Could you check a few things on this drawing? It's one solid part, dimensions in mm from its lowest x, y, z. A direction names the side the tool comes from. Coordinates: 2 decimals unless noted, no trailing zeros. Write each loop counter-clockwise with the first axis right and the second up, starting at its lowest first coordinate (ties: lowest second). Pieces come first, ordered by that corner, then holes. Notation, with made-up numbers: M -37,16.5 L 5,16.5 A23 ccw 5,47.5 Z; hole C -18.75,76.25 d10. An arc over 180 degrees is marked long. Use a Markdown table: item, result.
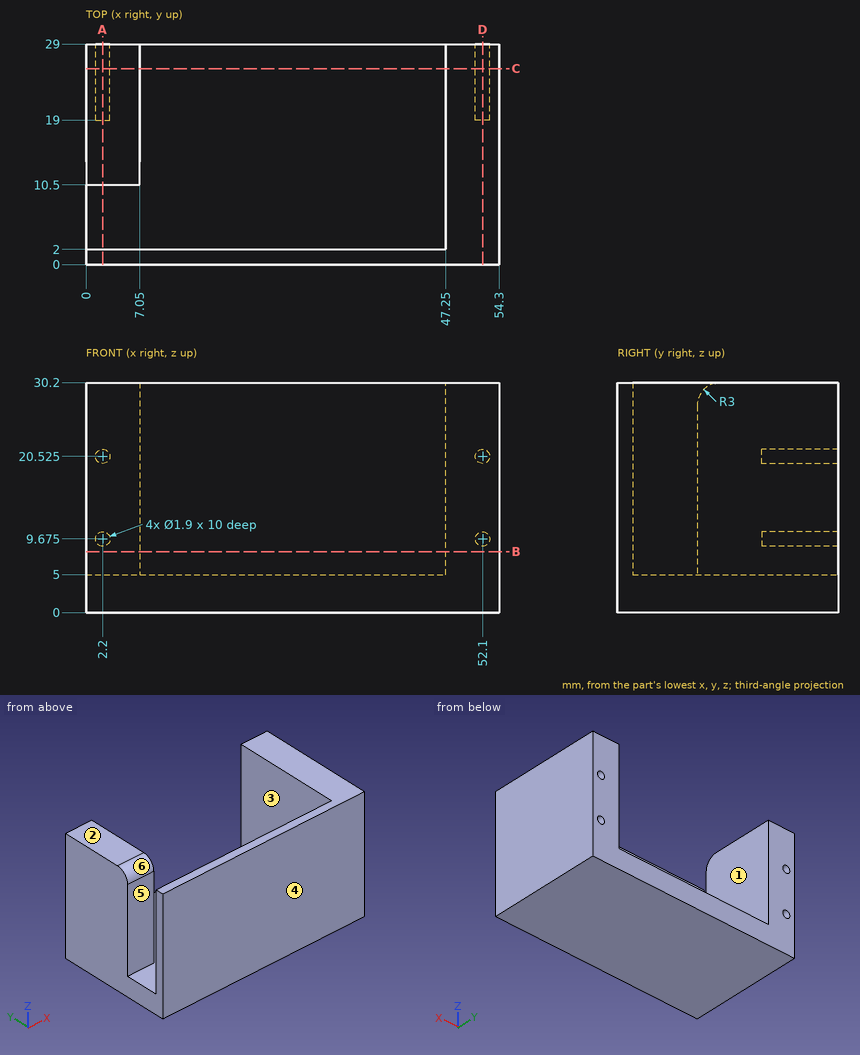
1. Which directions (+Z, -Z, +X, -X, +Y, -Y) give clear straight access to the entire face, cutting with the end or side of a thin tool? Please do the marked faces 1 and 2.
Answers follow:
| item | result |
|---|---|
| face 1 | +Z, +Y |
| face 2 | +Z, +X, -X, +Y, -Y |
2. Will these pins go through, and if not, where does the flat tip stop? pin 1 Ø6 at (x, y) = (25, 10.5) entering from +Z; pin 2 Ø0.9 at (x, z) = (52.5, 9.5) entering from +Y.
Answers follow:
| item | result |
|---|---|
| pin 1 | stops at z = 5 |
| pin 2 | stops at y = 19 |
3. Suppose I cut it at A-A on x = 2.2. Write out the boundary of the cut face in (y, z) (3 decimals), and give its area (3 significant figures).
Answers follow:
| item | result |
|---|---|
| outline | M 0,0 L 29,0 L 29,8.725 L 19,8.725 L 19,10.625 L 29,10.625 L 29,19.575 L 19,19.575 L 19,21.475 L 29,21.475 L 29,30.2 L 13.5,30.2 A3 ccw 10.5,27.2 L 10.5,5 L 2,5 L 2,30.2 L 0,30.2 Z |
| area | 622 mm2 |
4. Suppose I cut it at B-B on z = 8. Write out the boundary of the cut face in (x, y), and give its area (3 significant figures).
Answers follow:
| item | result |
|---|---|
| outline | M 0,0 L 54.3,0 L 54.3,29 L 47.25,29 L 47.25,2 L 0,2 Z; M 0,10.5 L 7.05,10.5 L 7.05,29 L 0,29 Z |
| area | 429 mm2 |
5. Suppose I cut it at D-D on x = 52.1. Write out the boundary of the cut face in (y, z) (3 decimals).
Answers follow:
| item | result |
|---|---|
| outline | M 0,0 L 29,0 L 29,8.725 L 19,8.725 L 19,10.625 L 29,10.625 L 29,19.575 L 19,19.575 L 19,21.475 L 29,21.475 L 29,30.2 L 0,30.2 Z |
6. Suppose I cut it at C-C on y = 25.75. Write out the boundary of the cut face in (x, z) (3 decimals), and give its area (3 significant figures).
Answers follow:
| item | result |
|---|---|
| outline | M 0,0 L 54.3,0 L 54.3,30.2 L 47.25,30.2 L 47.25,5 L 7.05,5 L 7.05,30.2 L 0,30.2 Z; hole C 2.2,9.675 d1.9; hole C 2.2,20.525 d1.9; hole C 52.1,9.675 d1.9; hole C 52.1,20.525 d1.9 |
| area | 615 mm2 |
7. I need wall thicknesses on probe 1 along Z at (x, y) = (52.1, 21.75) (3 decimals); probe 2 along X at (y, z) = (25, 15); probe 3 along Y at (x, z) = (20, 15.5). Which ranges of each line are inside material? Lowest first, please.
Answers follow:
| item | result |
|---|---|
| probe 1 | z = 0 to 8.725, 10.625 to 19.575, 21.475 to 30.2 |
| probe 2 | x = 0 to 7.05, 47.25 to 54.3 |
| probe 3 | y = 0 to 2 |
8. We'd pull the mould along Y, two halves only. Please class the marked faces 3, 4, 5 and 6: +Y half, -Y half, draft (parallel to the pull), parting line (faces both ways), or undercut.
Answers follow:
| item | result |
|---|---|
| face 3 | draft |
| face 4 | -Y half |
| face 5 | undercut |
| face 6 | undercut |
